Check sheet for the modelled part. Datum: model origin and axes. Units: mm. A direction names the side the tool comes from. Coordinates: 2 decimals unless noted, no trailing zeros. Order: outer loops, then holes, each group sorted by start corner. A loop starts at its lowest first (then second) coordinate and runs counter-clockwise, first axis right, second up. Notation, with made-up numbers: (21.25, 30) -> (51.25, 30) arc R36 ccw to (51.25, 65) -> close; hole circle Ø3 at (19, 10.25). An arc over 180 degrees is marked (long way). Put each result on its own line as item: value. Start each with the question number.
```python
from build123d import *

# Parameters (mm, degrees)
SKETCH3_W          = 400
SKETCH3_H          = 25
SKETCH5_R          = 20
CUT_EXTRUDE3_DEPTH = 403.550581854
SKETCH8_W          = 250
SKETCH8_H          = 31.237018092
CUT_EXTRUDE2_DEPTH = 78


with BuildPart() as part:
    # Sketch3 → Revolve1 (revolve)
    with BuildSketch(Plane.XY, mode=Mode.PRIVATE) as revolve1_sk:
        with Locations((27.926421405, 25.2090301)):
            Rectangle(SKETCH3_W, SKETCH3_H)
    revolve(revolve1_sk.sketch.rotate(Axis((-172.073578595, 12.7090301, 0), (1, 0, 0)), 90), axis=Axis((-172.073578595, 12.7090301, 0), (1, 0, 0)))

    # Sketch5 → Cut-Extrude3 (cut, through all)
    with BuildSketch(Plane.ZY.offset(172.073578595)):
        with Locations((0, 12.7090301)):
            Circle(SKETCH5_R)
    extrude(amount=-CUT_EXTRUDE3_DEPTH, mode=Mode.SUBTRACT)

    # Sketch8 → Cut-Extrude2 (cut)
    with BuildSketch(Plane(origin=(0, 100, 0), x_dir=(1, 0, 0), z_dir=(0, 1, 0))):
        with Locations((-27.073578595, 0)):
            Rectangle(SKETCH8_W, SKETCH8_H)
    extrude(amount=-CUT_EXTRUDE2_DEPTH, mode=Mode.SUBTRACT)


solid = part.part
```
1) Sectioned sample at A-A (z = 0). Record the boundary of the cut face in (x, y).
2) Gauge pin test, flat ends, axial feed: pin 1 (10 mm diameter, centred on x = -90.5, y = 2, fed in from -Z); pin 2 (4 mm diameter, centred on x = 138.5, y = 26, fed in from +Z) (3 decimals); pin 3 (3.5 mm diameter, centred on x = -38.5, y = 29, fed in from -Z); pin 4 (10 mm diameter, centred on y = 28, z = -8.5, fed in from -X). Record the tip position at first contact, or that the pin passes through.
3) Sectioned sample at C-C (x = 160.5). Record the boundary of the cut face in (y, z).
4) Sectioned sample at D-D (y = 28.5). Record the boundary of the cut face in (x, z).
5) Access from +Z, -Z, +X, -X, +Y, -Y to the whole of each face (thin tool, end or side, straight path). Record for faces 1 (the cylindrical face through (25.126, -5.034, 9.229)), 2 (the flat face through (-29, 29, -15.619)).
6) Scan lines: line 1 along X through (y, z) = (35, -7.5); line 2 along Y through (x, z) = (131, 0); line 3 along Z through (x, y) = (109, 6). Record each from-to range of solid material in increasing order. Write a range as [from, to].
7) Sectioned sample at B-B (y = 5). Record the boundary of the cut face in (x, z).
8) Mould release check, pull along X, two halves, no side actions. Record for faces 3 (the flat face through (-172.074, -4.1, 11.2)), 4 (the cylindrical face through (30.73, -12.08, -3.25)), 5 (the flat face through (-29, 29, 15.619)): +X half, -X half, draft (parallel to the pull), parting line (faces both ways), or undercut.
Entries:
1. outline: (-172.07, -12.29) -> (227.93, -12.29) -> (227.93, -7.29) -> (-172.07, -7.29) -> close; (-172.07, 32.71) -> (-152.07, 32.71) -> (-152.07, 37.71) -> (-172.07, 37.71) -> close; (97.93, 32.71) -> (227.93, 32.71) -> (227.93, 37.71) -> (97.93, 37.71) -> close
2. pin 1: stops at z = -24.34
2. pin 2: stops at z = 22.305
2. pin 3: stops at z = -20.34
2. pin 4: stops at x = -172.07
3. outline: circle Ø50 at (12.71, 0); hole circle Ø40 at (12.71, 0)
4. outline: (-172.07, -19.38) -> (227.93, -19.38) -> (227.93, -12.27) -> (97.93, -12.27) -> (97.93, -15.62) -> (-152.07, -15.62) -> (-152.07, -12.27) -> (-172.07, -12.27) -> close; (-172.07, 12.27) -> (-152.07, 12.27) -> (-152.07, 15.62) -> (97.93, 15.62) -> (97.93, 12.27) -> (227.93, 12.27) -> (227.93, 19.38) -> (-172.07, 19.38) -> close
5. face 1: +X, -X
5. face 2: +Y
6. line 1: x = [-172.07, -152.07], [97.93, 227.93]
6. line 2: y = [-12.29, -7.29], [32.71, 37.71]
6. line 3: z = [-24.08, -18.84], [18.84, 24.08]
7. outline: (-172.07, -23.78) -> (227.93, -23.78) -> (227.93, -18.45) -> (-172.07, -18.45) -> close; (-172.07, 18.45) -> (227.93, 18.45) -> (227.93, 23.78) -> (-172.07, 23.78) -> close
8. face 3: -X half
8. face 4: draft
8. face 5: undercut
